The listing builds one solid part. Answer for the finished solid, in the listing's coordinates (mm). Face numbers are marked on the shaded views. A direction names the side the tool comes from. Coordinates: 2 decimals unless noted, no trailing zeros. Loops run counter-clockwise (first coordinate to the right, second up) from the corner with the lowest first, then second, coordinate; pieces in that order, holes last. Notation, with made-up numbers: (-4, 48) - (18, 48) arc R10 ccw to (18, 64) - close; hole circle Ø1 at (14.25, 75.25). An arc over 180 degrees is marked (long way). Write each question's results on one line, items separated by ' | '. Start each with the question number.
(1) Given pin 1 Ø8 at (x, y) = (8, 7) entering from -Z; pin 2 Ø4 at (x, y) = (0, 0) entering from -Z; pin 3 Ø1 at (y, z) = (2, 9.5) entering from -X; pin 4 Ø4 at (y, z) = (11.5, 5) entering from +X, each flat-ended and moving along its own axis, determine where each tip first touches the part or whether it passes through.
(2) Find section C-C on x = 13. Determine the outline of the cut face in (y, z), then the cut area to 3 significant figures.
(3) Consider line 1 (Z direction, x = 7.5, y = 4.5); line 2 (Y direction, x = 22.5, z = 5.75); line 3 (Y direction, x = 0, z = 15.2). Determine where each line is inside the solid, lowest interval first. Write a range as from..to.
(4) Determine the mould class of the marked faces 5, 6 and 7 for opening direction Y: released by +Y, released by -Y, zero draft, split by the parting line, or undercut.
(5) Find section D-D on x = 3. Determine the outline of the cut face in (y, z), then the cut area to 3 significant figures.
(6) Find section B-B on z = 14.75. Determine the outline of the cut face in (x, y), then the cut area to 3 significant figures.
(7) For the marked faces 1, 2, 3 and 4, determine the directions among +Z, -Z, +X, -X, +Y, -Y from which every point of the face is accessible in a straight line to the end or side of a thin tool.
(8) Find section A-A on z = 7.25. State how many separate pieces and enclosed holes the cut face has, then the cut area to 3 significant figures.
from build123d import *

# Parameters (mm, degrees)
BOSS_EXTRUDE1_DEPTH  = 14.025885253
BOSS_EXTRUDE2_DEPTH  = 2.54
CIRPATTERN1_START    = 14.025885253
CIRPATTERN1_DEPTH    = 2.54
CIRPATTERN1_2_DEPTH  = 14.025885253
FILLET1_R            = 1.27
M4_CLEARANCE_HOLE1_D = 4.5


# Read off the part's stored shape, not the designer's step: CirPattern1
with BuildPart() as part:
    # Sketch1 → Boss-Extrude1 (new body)
    with BuildSketch(Plane.XY):
        with BuildLine():
            Line((-22.987, 16.701033091), (-22.987, 9.084847245))
            Line((-22.987, 9.084847245), (-21.59, 9.084847245))
            ThreePointArc((-21.59, 9.084847245), (-20.982965782, 9.25936469), (-20.5613, 9.729625096))
            Line((-20.5613, 9.729625096), (-20.447, 9.965625061))
            Line((-20.447, 9.965625061), (-20.447, 14.85561507))
            Line((-20.447, 14.85561507), (-15.796343137, 16.366705085))
            Line((-15.796343137, 16.366705085), (-15.607214475, 16.548338845))
            ThreePointArc((-15.607214475, 16.548338845), (-15.290272145, 17.094685292), (-15.31188008, 17.725937997))
            Line((-15.31188008, 17.725937997), (-15.743576822, 19.05456395))
            Line((-15.743576822, 19.05456395), (-22.987, 16.701033091))
        make_face()
    extrude(amount=BOSS_EXTRUDE1_DEPTH)

    # Sketch2 → Boss-Extrude2 (add)
    with BuildSketch(Plane.XY.offset(14.025885253)):
        with BuildLine():
            Line((-22.987, 9.084847245), (-6.980044584, -2.544886608))
            ThreePointArc((-6.980044584, -2.544886608), (6.01059176, -4.366950532), (0.263378594, 7.424830097))
            Line((0.263378594, 7.424830097), (-15.743576822, 19.05456395))
            Line((-15.743576822, 19.05456395), (-22.987, 16.701033091))
            Line((-22.987, 16.701033091), (-22.987, 9.084847245))
        make_face()
    extrude(amount=BOSS_EXTRUDE2_DEPTH)

    # CirPattern1 outline → CirPattern1 (add)
    with BuildSketch(Plane.XY.offset(CIRPATTERN1_START)):
        with BuildLine():
            Line((-10.482780502, 0), (-22.987, -9.084847245))
            Line((-22.987, -9.084847245), (-22.987, -16.701033091))
            Line((-22.987, -16.701033091), (-15.743576822, -19.05456395))
            Line((-15.743576822, -19.05456395), (0.263378594, -7.424830097))
            ThreePointArc((0.263378594, -7.424830097), (-4.151127873, -6.161623782), (-6.980044584, -2.544886608))
            Line((-6.980044584, -2.544886608), (-10.482780502, 0))
        make_face()
        with BuildLine():
            ThreePointArc((4.151127873, 6.161623782), (7.4295, 0), (4.151127873, -6.161623782))
            Line((4.151127873, -6.161623782), (23.93681288, -6.161623782))
            Line((23.93681288, -6.161623782), (28.413494599, 0))
            Line((28.413494599, 0), (23.93681288, 6.161623782))
            Line((23.93681288, 6.161623782), (4.151127873, 6.161623782))
        make_face()
    extrude(amount=CIRPATTERN1_DEPTH)

    # CirPattern1 2 outline → CirPattern1 2 (add)
    with BuildSketch(Plane.XY):
        with BuildLine():
            Line((-20.447, -14.85561507), (-20.447, -9.965625061))
            Line((-20.447, -9.965625061), (-20.5613, -9.729625096))
            ThreePointArc((-20.5613, -9.729625096), (-20.982965782, -9.25936469), (-21.59, -9.084847245))
            Line((-21.59, -9.084847245), (-22.987, -9.084847245))
            Line((-22.987, -9.084847245), (-22.987, -16.701033091))
            Line((-22.987, -16.701033091), (-15.743576822, -19.05456395))
            Line((-15.743576822, -19.05456395), (-15.31188008, -17.725937997))
            ThreePointArc((-15.31188008, -17.725937997), (-15.290272145, -17.094685292), (-15.607214475, -16.548338845))
            Line((-15.607214475, -16.548338845), (-15.796343137, -16.366705085))
            Line((-15.796343137, -16.366705085), (-20.447, -14.85561507))
        make_face()
        with BuildLine():
            Line((22.806616138, -5.340487785), (23.93681288, -6.161623782))
            Line((23.93681288, -6.161623782), (28.413494599, 0))
            Line((28.413494599, 0), (23.93681288, 6.161623782))
            Line((23.93681288, 6.161623782), (22.806616138, 5.340487785))
            ThreePointArc((22.806616138, 5.340487785), (22.418093921, 4.842494444), (22.353371268, 4.214196857))
            Line((22.353371268, 4.214196857), (22.399617925, 3.95608502))
            Line((22.399617925, 3.95608502), (25.273881936, 0))
            Line((25.273881936, 0), (22.399617925, -3.95608502))
            Line((22.399617925, -3.95608502), (22.353371268, -4.214196857))
            ThreePointArc((22.353371268, -4.214196857), (22.418093921, -4.842494444), (22.806616138, -5.340487785))
        make_face()
    extrude(amount=CIRPATTERN1_2_DEPTH)

    # Fillet1
    fillet1_edges = [part.edges().sort_by_distance(p)[0] for p in [
        (-10.482780502, 0, 15.295885253),
    ]]
    fillet(fillet1_edges, radius=FILLET1_R)

    # M4 Clearance Hole1 (through all)
    with Locations(Plane.XY.offset(16.565885253)):
        with Locations((0, 0)):
            Hole(M4_CLEARANCE_HOLE1_D / 2)


solid = part.part
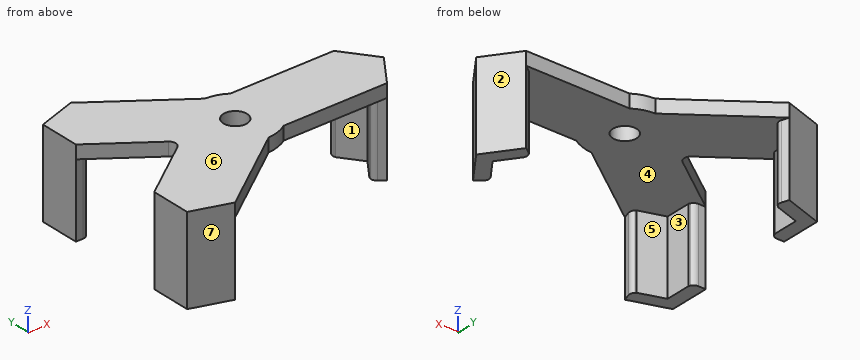
Values:
1) pin 1: stops at z = 14.03 | pin 2: passes through | pin 3: stops at x = 23.46 | pin 4: stops at x = -20.45
2) outline: (-6.16, 14.03) - (6.16, 14.03) - (6.16, 16.57) - (-6.16, 16.57) - close | area: 31.3 mm²
3) line 1: z = 14.03..16.57 | line 2: y = -5.01..-3.82, 3.82..5.01 | line 3: y = -7.62..-2.25, 2.25..7.62
4) face 5: undercut | face 6: zero draft | face 7: released by -Y
5) outline: (-6.8, 14.03) - (6.8, 14.03) - (6.8, 16.57) - (-6.8, 16.57) - close | area: 34.5 mm²
6) outline: (-22.99, -16.7) - (-15.74, -19.05) - (0.26, -7.42) arc R7.43 ccw to (4.15, -6.16) - (23.94, -6.16) - (28.41, 0) - (23.94, 6.16) - (4.15, 6.16) arc R7.43 ccw to (0.26, 7.42) - (-15.74, 19.05) - (-22.99, 16.7) - (-22.99, 9.08) - (-11.9, 1.03) arc R1.27 cw to (-11.9, -1.03) - (-22.99, -9.08) - close; hole circle Ø4.5 at (0, 0) | area: 880 mm²
7) face 1: -Z, -X | face 2: +Z, -Z, +X, +Y | face 3: -Z, +X | face 4: -Z
8) separate pieces: 3 | enclosed holes: 0 | area: 100 mm²
